from build123d import *

# Parameters (mm, degrees)
F1_DEPTH = 6.35


with BuildPart() as f1:
    # F0 (on Front) → F1 (new body)
    with BuildSketch(Plane.XZ):
        with BuildLine():
            Line((0.222685, 19.048698), (-203.471396, 21.429948))
            ThreePointArc((-203.471396, 21.429948), (-222.74278, 2.603935), (-203.916767, -16.667448))
            Line((-203.916767, -16.667448), (-0.222685, -19.048698))
            ThreePointArc((-0.222685, -19.048698), (19.048698, -0.222685), (0.222685, 19.048698))
        make_face()
        with BuildLine():
            Line((-0.176293, -15.08022), (-203.870374, -12.69897))
            ThreePointArc((-203.870374, -12.69897), (-218.774301, 2.557543), (-203.517789, 17.46147))
            Line((-203.517789, 17.46147), (0.176293, 15.08022))
            ThreePointArc((0.176293, 15.08022), (15.08022, -0.176293), (-0.176293, -15.08022))
        make_face(mode=Mode.SUBTRACT)
    extrude(amount=F1_DEPTH)


solid = f1.part
Design review of the part built by this model. Coordinates are the model's own, in mm. Round coordinates to 2 decimals unless told otherwise and drop trailing zeros. Write each loop counter-clockwise with the first axis right and the second up, starting at its lowest first coordinate (ties: lowest second). Pieces come first, ordered by that corner, then holes.
Item 1: Consider section B-B on z = 1.5. Give the boundary of the cut face in (x, y), and give its area (3 significant figures).
Item 2: Consider section A-A on y = -5. Give the boundary of the cut face in (x, z), and give its area (3 significant figures).
Item 3: Consider section C-C on x = -62.5. Give the boundary of the cut face in (y, z).
Item 4: For pin 1 Ø4 at (x, z) = (-110, 12.5) entering from +Y, flat-tipped, find the tip position at first contact; note if it passes through.
Item 5: Wall thickness on L1, parallel to Z at x = -96, y = -2; L2, parallel to X at y = -2.25, z = 10; L3, parallel to Z at x = -120.5, y = -0.75: over which ranges is each line inside the solid? List them lowest first.
Item 6: Draft analysis for pull direction Z (two halves, no side actions). For faces 1 (the cylindrical face through (15.08, -3.13, 0.16)), 2 (the cylindrical face through (-222.733, -3.131, 3.023)), 3 (the cylindrical face through (-218.775, -3.131, 2.226)), 4 (the flat face through (-111, -6.35, -15)), state which applies: released by +Z, released by -Z, zero draft, split by the parting line, or undercut.
Check values:
1. outline: (-222.72, -6.35) - (-218.75, -6.35) - (-218.75, 0) - (-222.72, 0) - close; (15.01, -6.35) - (18.99, -6.35) - (18.99, 0) - (15.01, 0) - close
1. area: 50.5 mm2
2. outline: (-203.92, -16.67) - (-0.22, -19.05) arc R19.05 ccw to (0.22, 19.05) - (-203.47, 21.43) arc R19.05 ccw to start; hole (-203.87, -12.7) - (-0.18, -15.08) arc R15.08 ccw to (0.18, 15.08) - (-203.52, 17.46) arc R15.08 ccw to start
2. area: 2,040 mm2
3. outline: (-6.35, -18.32) - (0, -18.32) - (0, -14.35) - (-6.35, -14.35) - close; (-6.35, 15.81) - (0, 15.81) - (0, 19.78) - (-6.35, 19.78) - close
4. pin 1: passes through
5. L1: z = -17.93 to -13.96, 16.2 to 20.17
5. L2: x = -221.15 to -216.71, 11.29 to 16.21
5. L3: z = -17.64 to -13.67, 16.49 to 20.46
6. face 1: undercut
6. face 2: split by the parting line
6. face 3: undercut
6. face 4: zero draft
